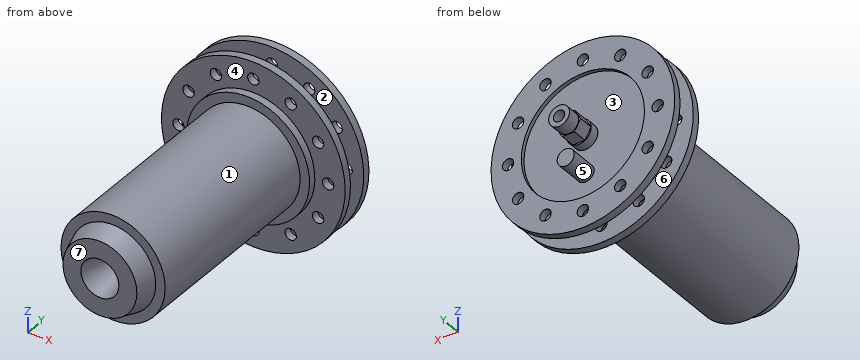
```python
from build123d import *

# Parameters (mm, degrees)
SKETCH_2_W                = 16
SKETCH_2_H                = 4
SKETCH_3_R                = 3
CUT_EXTRUDE_1_DEPTH       = 10
PATTERN_CIRCULAR_1_COUNT  = 12
MIRROR_2_COPY_1_SKETCH_R  = 3
MIRROR_2_COPY_1_DEPTH     = 10
MIRROR_2_COPY_2_SKETCH_R  = 3
MIRROR_2_COPY_2_DEPTH     = 10
MIRROR_2_COPY_3_SKETCH_R  = 3
MIRROR_2_COPY_3_DEPTH     = 10
MIRROR_2_COPY_4_SKETCH_R  = 3
MIRROR_2_COPY_4_DEPTH     = 10
MIRROR_2_COPY_5_SKETCH_R  = 3
MIRROR_2_COPY_5_DEPTH     = 10
MIRROR_2_COPY_6_SKETCH_R  = 3
MIRROR_2_COPY_6_DEPTH     = 10
MIRROR_2_COPY_7_SKETCH_R  = 3
MIRROR_2_COPY_7_DEPTH     = 10
MIRROR_2_COPY_8_SKETCH_R  = 3
MIRROR_2_COPY_8_DEPTH     = 10
MIRROR_2_COPY_9_SKETCH_R  = 3
MIRROR_2_COPY_9_DEPTH     = 10
MIRROR_2_COPY_10_SKETCH_R = 3
MIRROR_2_COPY_10_DEPTH    = 10
MIRROR_2_COPY_11_SKETCH_R = 3
MIRROR_2_COPY_11_DEPTH    = 10
CUT_EXTRUDE_2_DEPTH       = 8
SKETCH_7_W                = 4.5
SKETCH_7_H                = 15


with BuildPart() as part:
    # Эскиз1 → Повернуть1 (revolve)
    with BuildSketch(Plane.XY, mode=Mode.PRIVATE) as revolve_1_sk:
        Polygon((10, 0), (19.5, 0), (22.5, 10), (27.5, 10), (27.5, 112), (32.5, 112), (32.5, 120), (35, 120), (35, 130), (32.5, 130), (32.5, 132), (0, 132), (0, 20), (5, 20), align=None)
    revolve(revolve_1_sk.sketch.rotate(Axis((0, 0, 0), (0, 1, 0)), 90), axis=Axis((0, 0, 0), (0, 1, 0)))

    # Эскиз2 → Повернуть2 (revolve)
    with BuildSketch(Plane(origin=(0, 0, 0), x_dir=(0, 0, -1), z_dir=(1, 0, 0))):
        with Locations((40.5, 118)):
            Rectangle(SKETCH_2_W, SKETCH_2_H)
    revolve_2 = revolve(axis=Axis((0, 0, 0), (0, 1, 0)))

    # Эскиз3 → Вырез-Вытянуть1 (cut)
    with BuildSketch(Plane(origin=(0, 120, 0), x_dir=(1, 0, 0), z_dir=(0, 1, 0))):
        with Locations(Location((39.5, 0, 0), (0, 0, 270))):
            Circle(SKETCH_3_R)
    cut_extrude_1 = extrude(amount=-CUT_EXTRUDE_1_DEPTH, mode=Mode.SUBTRACT)

    # Круговой массив1: Вырез-Вытянуть1 ×12 about axis
    pattern_circular_1_axis = Axis((0, 0, 0), (0, 1, 0))
    for i in range(1, PATTERN_CIRCULAR_1_COUNT):
        add(cut_extrude_1.rotate(pattern_circular_1_axis, i * 360 / PATTERN_CIRCULAR_1_COUNT), mode=Mode.SUBTRACT)

    # Зеркальное отражение2: Повернуть2, Вырез-Вытянуть1 across plane
    add(revolve_2.mirror(Plane.ZX.offset(125)))
    add(cut_extrude_1.mirror(Plane.ZX.offset(125)), mode=Mode.SUBTRACT)

    # Зеркальное отражение2 copy 1 sketch → Зеркальное отражение2 copy 1 (cut)
    with BuildSketch(Plane(origin=(0, 130, 0), x_dir=(0.8660254037844387, 0, -0.49999999999999994), z_dir=(0, -1, 0))):
        with Locations((39.5, 0)):
            Circle(MIRROR_2_COPY_1_SKETCH_R)
    extrude(amount=-MIRROR_2_COPY_1_DEPTH, mode=Mode.SUBTRACT)

    # Зеркальное отражение2 copy 2 sketch → Зеркальное отражение2 copy 2 (cut)
    with BuildSketch(Plane(origin=(0, 130, 0), x_dir=(0.5000000000000001, 0, -0.8660254037844386), z_dir=(0, -1, 0))):
        with Locations((39.5, 0)):
            Circle(MIRROR_2_COPY_2_SKETCH_R)
    extrude(amount=-MIRROR_2_COPY_2_DEPTH, mode=Mode.SUBTRACT)

    # Зеркальное отражение2 copy 3 sketch → Зеркальное отражение2 copy 3 (cut)
    with BuildSketch(Plane(origin=(0, 130, 0), x_dir=(0, 0, -1), z_dir=(0, -1, 0))):
        with Locations((39.5, 0)):
            Circle(MIRROR_2_COPY_3_SKETCH_R)
    extrude(amount=-MIRROR_2_COPY_3_DEPTH, mode=Mode.SUBTRACT)

    # Зеркальное отражение2 copy 4 sketch → Зеркальное отражение2 copy 4 (cut)
    with BuildSketch(Plane(origin=(0, 130, 0), x_dir=(-0.4999999999999998, 0, -0.8660254037844387), z_dir=(0, -1, 0))):
        with Locations((39.5, 0)):
            Circle(MIRROR_2_COPY_4_SKETCH_R)
    extrude(amount=-MIRROR_2_COPY_4_DEPTH, mode=Mode.SUBTRACT)

    # Зеркальное отражение2 copy 5 sketch → Зеркальное отражение2 copy 5 (cut)
    with BuildSketch(Plane(origin=(0, 130, 0), x_dir=(-0.8660254037844387, 0, -0.49999999999999994), z_dir=(0, -1, 0))):
        with Locations((39.5, 0)):
            Circle(MIRROR_2_COPY_5_SKETCH_R)
    extrude(amount=-MIRROR_2_COPY_5_DEPTH, mode=Mode.SUBTRACT)

    # Зеркальное отражение2 copy 6 sketch → Зеркальное отражение2 copy 6 (cut)
    with BuildSketch(Plane(origin=(0, 130, 0), x_dir=(-1, 0, 0), z_dir=(0, -1, 0))):
        with Locations((39.5, 0)):
            Circle(MIRROR_2_COPY_6_SKETCH_R)
    extrude(amount=-MIRROR_2_COPY_6_DEPTH, mode=Mode.SUBTRACT)

    # Зеркальное отражение2 copy 7 sketch → Зеркальное отражение2 copy 7 (cut)
    with BuildSketch(Plane(origin=(0, 130, 0), x_dir=(-0.8660254037844386, 0, 0.5000000000000001), z_dir=(0, -1, 0))):
        with Locations((39.5, 0)):
            Circle(MIRROR_2_COPY_7_SKETCH_R)
    extrude(amount=-MIRROR_2_COPY_7_DEPTH, mode=Mode.SUBTRACT)

    # Зеркальное отражение2 copy 8 sketch → Зеркальное отражение2 copy 8 (cut)
    with BuildSketch(Plane(origin=(0, 130, 0), x_dir=(-0.5000000000000004, 0, 0.8660254037844384), z_dir=(0, -1, 0))):
        with Locations((39.5, 0)):
            Circle(MIRROR_2_COPY_8_SKETCH_R)
    extrude(amount=-MIRROR_2_COPY_8_DEPTH, mode=Mode.SUBTRACT)

    # Зеркальное отражение2 copy 9 sketch → Зеркальное отражение2 copy 9 (cut)
    with BuildSketch(Plane(origin=(0, 130, 0), x_dir=(0, 0, 1), z_dir=(0, -1, 0))):
        with Locations((39.5, 0)):
            Circle(MIRROR_2_COPY_9_SKETCH_R)
    extrude(amount=-MIRROR_2_COPY_9_DEPTH, mode=Mode.SUBTRACT)

    # Зеркальное отражение2 copy 10 sketch → Зеркальное отражение2 copy 10 (cut)
    with BuildSketch(Plane(origin=(0, 130, 0), x_dir=(0.5000000000000001, 0, 0.8660254037844386), z_dir=(0, -1, 0))):
        with Locations((39.5, 0)):
            Circle(MIRROR_2_COPY_10_SKETCH_R)
    extrude(amount=-MIRROR_2_COPY_10_DEPTH, mode=Mode.SUBTRACT)

    # Зеркальное отражение2 copy 11 sketch → Зеркальное отражение2 copy 11 (cut)
    with BuildSketch(Plane(origin=(0, 130, 0), x_dir=(0.8660254037844384, 0, 0.5000000000000004), z_dir=(0, -1, 0))):
        with Locations((39.5, 0)):
            Circle(MIRROR_2_COPY_11_SKETCH_R)
    extrude(amount=-MIRROR_2_COPY_11_DEPTH, mode=Mode.SUBTRACT)

    # Эскиз4 → Повернуть3 (revolve)
    with BuildSketch(Plane(origin=(0, 0, 0), x_dir=(0, 0, -1), z_dir=(1, 0, 0))):
        Polygon((6.5, 132), (6.5, 145), (5.5, 145), (5.5, 152), (3, 152), (3, 132), align=None)
    revolve(axis=Axis((0, 0, 0), (0, 1, 0)))

    # Эскиз5 → Вырез-Вытянуть2 (cut)
    with BuildSketch(Plane(origin=(0, 145, 0), x_dir=(1, 0, 0), z_dir=(0, 1, 0))):
        with BuildLine():
            Line((-3.25, 5.629165125), (3.25, 5.629165125))
            ThreePointArc((3.25, 5.629165125), (0, 6.5), (-3.25, 5.629165125))
        make_face()
        with BuildLine():
            Line((3.25, 5.629165125), (6.5, 0))
            ThreePointArc((6.5, 0), (5.629165125, 3.25), (3.25, 5.629165125))
        make_face()
        with BuildLine():
            ThreePointArc((3.25, -5.629165125), (5.629165125, -3.25), (6.5, 0))
            Line((6.5, 0), (3.25, -5.629165125))
        make_face()
        with BuildLine():
            ThreePointArc((-3.25, -5.629165125), (0, -6.5), (3.25, -5.629165125))
            Line((3.25, -5.629165125), (-3.25, -5.629165125))
        make_face()
        with BuildLine():
            ThreePointArc((-6.5, 0), (-5.629165125, -3.25), (-3.25, -5.629165125))
            Line((-3.25, -5.629165125), (-6.5, 0))
        make_face()
        with BuildLine():
            Line((-6.5, 0), (-3.25, 5.629165125))
            ThreePointArc((-3.25, 5.629165125), (-5.629165125, 3.25), (-6.5, 0))
        make_face()
    extrude(amount=-CUT_EXTRUDE_2_DEPTH, mode=Mode.SUBTRACT)

    # Эскиз7 → Повернуть5 (revolve)
    with BuildSketch(Plane(origin=(0, 0, 0), x_dir=(0, 0, -1), z_dir=(1, 0, 0))):
        with Locations((21.25, 139.5)):
            Rectangle(SKETCH_7_W, SKETCH_7_H)
    revolve(axis=Axis((0, 132, -19), (0, 1, 0)))


solid = part.part
```
Part model, mm, in its own coordinate system. Face numbers are marked on the shaded views. A direction names the side the tool comes from. Give positions to 0.01 mm unless a question says otherwise; leave off trailing zeros. Order: outer loops, then holes, each group sorted by start corner. A loop starts at its lowest first (then second) coordinate and runs counter-clockwise, first axis right, second up. Notation, with made-up numbers: (16.5, 40) - (58.5, 40) arc R28 ccw to (58.5, 72) - close; hole circle Ø2 at (86, 3.5). An arc over 180 degrees is marked (long way). Use one line per item in the form item = value.
Item 1: Slice it at B-B on x = 0. Count the separate pieces of the cut face and the enclosed holes in it, and give its area (3 significant figures).
Solution:
separate_pieces = 5
enclosed_holes = 0
area = 7,490 mm2
Item 2: Pin check, flat tips, straight feed: pin 1 Ø3.5 at (x, z) = (-39.5, 0) entering from -Y; pin 2 Ø8 at (x, z) = (35, -31.5) entering from +Y; pin 3 Ø8 at (y, z) = (58.5, -24.5) entering from -X; pin 4 Ø1.6 at (x, z) = (5.5, 2) entering from +Y. Stop position of each tip, or through.
Solution:
pin_1 = through
pin_2 = 134
pin_3 = -18.33
pin_4 = 152
Item 3: Probe probe 1 along X at (y, z) = (132.9, 0); probe 2 along X at (y, z) = (117.35, 0). List the from-to ranges inside material, lowest first. Write a range as from..to.
Solution:
probe_1 = -48.5..-42.5, -36.5..-32.5, -6.5..-3, 3..6.5, 32.5..36.5, 42.5..48.5
probe_2 = -48.5..-42.5, -36.5..36.5, 42.5..48.5
Item 4: Slice it at C-C on y = 17. Give the cut face in (x, z).
Solution:
outline = circle Ø55 at (0, 0); hole circle Ø11.5 at (0, 0)
Item 5: Slice it at A-A on z = 39.5. Give the cut face in (x, y).
Solution:
outline = (-28.14, 116) - (-3, 116) - (-3, 120) - (-28.14, 120) - close; (-28.14, 130) - (-3, 130) - (-3, 134) - (-28.14, 134) - close; (3, 116) - (28.14, 116) - (28.14, 120) - (3, 120) - close; (3, 130) - (28.14, 130) - (28.14, 134) - (3, 134) - close
Item 6: Slice it at D-D on x = 39.5. Give the cut face in (y, z), and give its area (3 significant figures).
Solution:
outline = (116, -28.14) - (120, -28.14) - (120, -3) - (116, -3) - close; (116, 3) - (120, 3) - (120, 28.14) - (116, 28.14) - close; (130, -28.14) - (134, -28.14) - (134, -3) - (130, -3) - close; (130, 3) - (134, 3) - (134, 28.14) - (130, 28.14) - close
area = 402 mm2
Item 7: Which spindle directions (+Z, -Z, +X, -X, +Y, -Y) get a long thin tool onto all of the face, cutting with end or side? Do the marked faces 4, 5, 6 and 7. Say none if no direction does.
Solution:
face_4 = -Y
face_5 = +Y
face_6 = none
face_7 = +Z, -Z, +X, -X, -Y
Item 8: Two-plate mould, pull along X, no slides. Class the marked faces 1, 2 and 3: released by +X, released by -X, zero draft, split by the parting line, or undercut.
Solution:
face_1 = split by the parting line
face_2 = zero draft
face_3 = undercut
